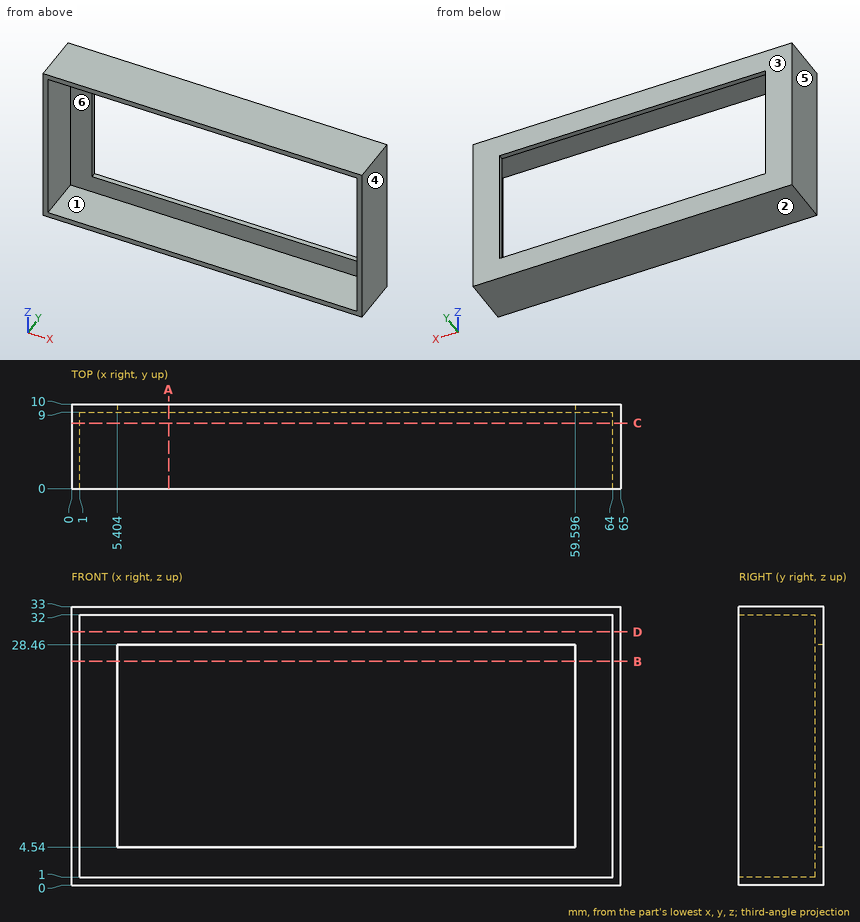
Check sheet for the drawn part. Datum: minimum x, y, z corner. Units: mm. A direction names the side the tool comes from. Round coordinates to 2 decimals unless told otherwise and drop trailing zeros. Order: outer loops, then holes, each group sorted by start corner. A loop starts at its lowest first (then second) coordinate and runs counter-clockwise, first axis right, second up.
1. Section check C-C on y = 7.75. Record the cut outline in (x, z), then the cut area to 3 significant figures.
Final values:
outline: (0, 0) - (65, 0) - (65, 33) - (0, 33) - close; hole (1, 1) - (64, 1) - (64, 32) - (1, 32) - close
area: 192 mm2
2. Access from +Z, -Z, +X, -X, +Y, -Y to the whole of each face (thin tool, end or side, straight path). Record for the marked faces 1 and 2.
Final values:
face 1: -Y
face 2: -Z, +X, -X, +Y, -Y
3. Release check for a two-part mould opening along X. For the marked faces 3, 4, 5 and 6 record: +X half, -X half, draft (parallel to the pull), parting line (faces both ways), or undercut.
Final values:
face 3: draft
face 4: +X half
face 5: -X half
face 6: undercut
4. Thickness scan on L1, parallel to Z at x = 17, y = 2.5; L2, parallel to X at y = 3.5, z = 14.5; L3, parallel to X at y = 9.25, z = 25. Record the ranges inside material, lowest first.
Final values:
L1: z = 0 to 1, 32 to 33
L2: x = 0 to 1, 64 to 65
L3: x = 0 to 5.4, 59.6 to 65
5. Section check D-D on z = 30. Record the cut outline in (x, y), then the cut area to 3 significant figures.
Final values:
outline: (0, 0) - (1, 0) - (1, 9) - (64, 9) - (64, 0) - (65, 0) - (65, 10) - (0, 10) - close
area: 83.0 mm2
6. Go/stop test with a flat-tipped pin: P1, Ø9.5, axis at x = 42, z = 12, coming from the -Y side. Record where the tip stops, or that it passes through.
Final values:
P1: passes through
7. Section check A-A on x = 11.5. Record the cut outline in (y, z), then the cut area to 3 significant figures.
Final values:
outline: (0, 0) - (10, 0) - (10, 4.54) - (9, 4.54) - (9, 1) - (0, 1) - close; (0, 32) - (9, 32) - (9, 28.46) - (10, 28.46) - (10, 33) - (0, 33) - close
area: 27.1 mm2
8. Section check B-B on z = 26.5. Record the cut outline in (x, y).
Final values:
outline: (0, 0) - (1, 0) - (1, 9) - (5.4, 9) - (5.4, 10) - (0, 10) - close; (59.6, 9) - (64, 9) - (64, 0) - (65, 0) - (65, 10) - (59.6, 10) - close
